Here's the drawing with two shaded views (mm, measured from the low corner). I have some questions. A direction names the side the tool comes from. Round coordinates to 2 decimals unless told otherwise and drop trailing zeros. Order: outer loops, then holes, each group sorted by start corner. A loop starts at its lowest first (then second) coordinate and runs counter-clockwise, first axis right, second up. Notation, with made-up numbers: (73.25, 78.25) -> (80.25, 78.25) arc R8 cw to (80.25, 82.25) -> close; hole circle Ø6 at (-14.75, -28). An arc over 180 degrees is marked (long way). Use a Markdown table: item, result. Add a question column.
Q1. If we section it at D-D on y = 35: List the corners of the cut face in (x, z) for me, plus the area to 3 significant figures.
Q2. I'm going to push flat-ended pins straight in: pin 1 Ø3 at (x, y) = (4, 35) entering from +Z; pin 2 Ø4.5 at (x, y) = (35.5, 2.5) entering from -Z; pin 3 Ø3 at (x, y) = (22.5, 13.5) entering from +Z. Where does each tip first touch, or does it pass through?
Q3. For the marked faces 1, 2 and 3, which set-ups out of +Z, -Z, +X, -X, +Y, -Y let a thin tool reach every point of the face, with its end or its side?
Q4. If we section it at B-B on x = 16: List the corners of the cut face in (y, z) for me, plus the area to 3 significant figures.
Q5. I need wall thicknesses on line 1 along X through (y, z) = (22, 3.75); line 2 along Z through (x, y) = (6, 36.5). Which ranges of each line are inside material? Lowest first, please. Write a range as [from, to].
Q6. If we section it at A-A on z = 2.75: List the corners of the cut face in (x, y) for me.
Q7. We'd pull the mould along X, two halves only. Please class the marked faces 4, 5 and 6: +X half, -X half, draft (parallel to the pull), parting line (faces both ways), or undercut.
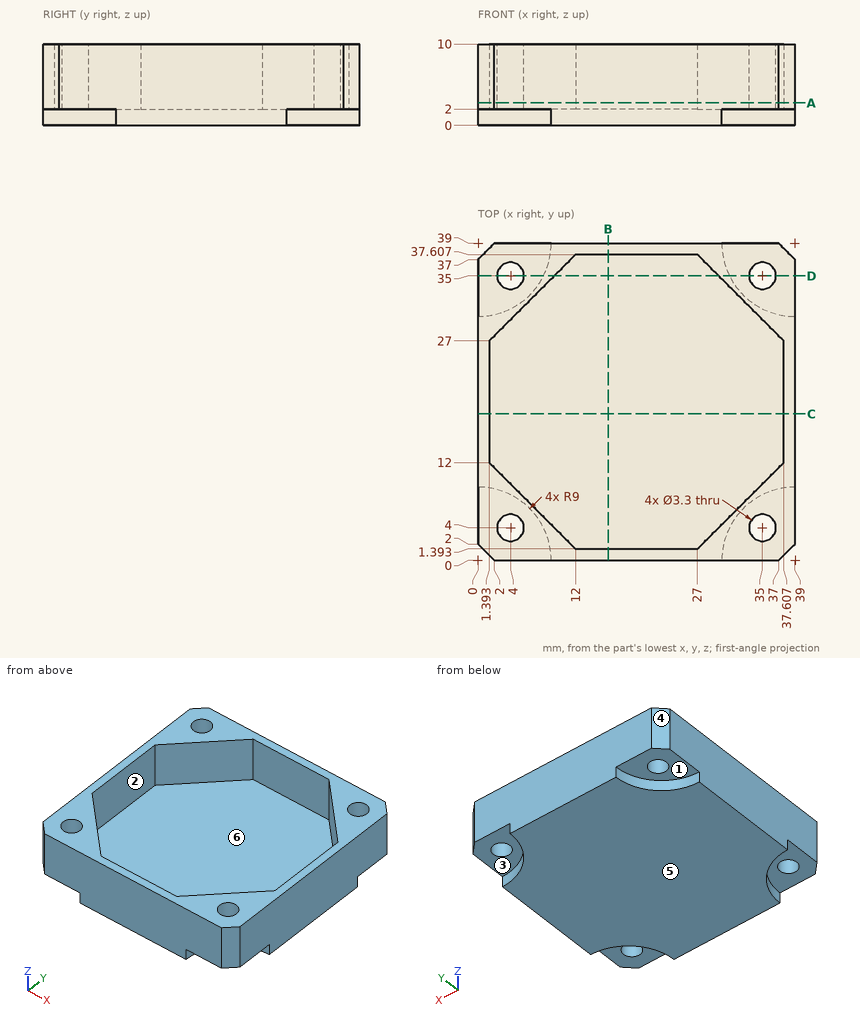
Answer below:
| question | item | result |
|---|---|---|
| 1 | outline | (0, 2) -> (2.35, 2) -> (2.35, 10) -> (0, 10) -> close; (5.65, 2) -> (8.06, 2) -> (8.06, 0) -> (30.94, 0) -> (30.94, 2) -> (33.35, 2) -> (33.35, 10) -> (29.61, 10) -> (29.61, 2) -> (9.39, 2) -> (9.39, 10) -> (5.65, 10) -> close; (36.65, 2) -> (39, 2) -> (39, 10) -> (36.65, 10) -> close |
| 1 | area | 143 mm² |
| 2 | pin 1 | through |
| 2 | pin 2 | z = 2 |
| 2 | pin 3 | z = 2 |
| 3 | face 1 | -Z, -X, +Y |
| 3 | face 2 | +Z |
| 3 | face 3 | -Z, +X, +Y |
| 4 | outline | (0, 0) -> (39, 0) -> (39, 10) -> (37.61, 10) -> (37.61, 2) -> (1.39, 2) -> (1.39, 10) -> (0, 10) -> close |
| 4 | area | 100 mm² |
| 5 | line 1 | [0, 1.39], [37.61, 39] |
| 5 | line 2 | [2, 10] |
| 6 | outline | (0, 2) -> (2, 0) -> (37, 0) -> (39, 2) -> (39, 37) -> (37, 39) -> (2, 39) -> (0, 37) -> close; hole (1.39, 12) -> (12, 1.39) -> (27, 1.39) -> (37.61, 12) -> (37.61, 27) -> (27, 37.61) -> (12, 37.61) -> (1.39, 27) -> close; hole circle Ø3.3 at (4, 4); hole circle Ø3.3 at (4, 35); hole circle Ø3.3 at (35, 4); hole circle Ø3.3 at (35, 35) |
| 7 | face 4 | -X half |
| 7 | face 5 | draft |
| 7 | face 6 | undercut |
